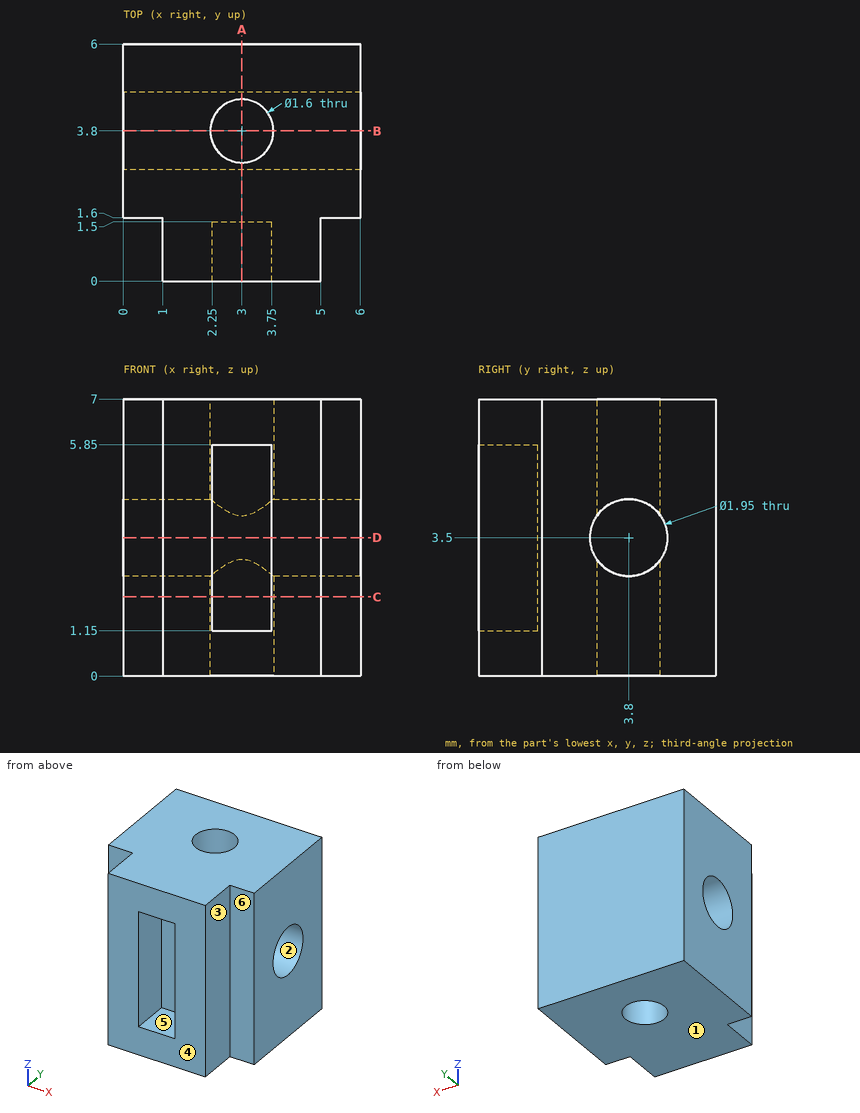
Design review of the part shown in the three views and the two pictorial views. Dimensions are in mm from the part's minimum x, y and z. A direction names the side the tool comes from. Round coordinates to 2 decimals unless told otherwise and drop trailing zeros. Order: outer loops, then holes, each group sorted by start corner. A loop starts at its lowest first (then second) coordinate and runs counter-clockwise, first axis right, second up.
Q1. Machinability: for the marked faces 4, 5 and 6, which of the approach directions +Z, -Z, +X, -X, +Y, -Y give a long, thin tool a straight path to every point of the face, cutting with its end or side? Answer none if there is none.
Findings below:
face 4: +Z, -Z, +X, -X, -Y
face 5: -Y
face 6: +Z, -Z, +X, -Y
Q2. We need section D-D, the plane z = 3.5. Give the boundary of the cut face in (x, y) (3 decimals).
Findings below:
outline: (0, 1.6) - (1, 1.6) - (1, 0) - (2.25, 0) - (2.25, 1.5) - (3.75, 1.5) - (3.75, 0) - (5, 0) - (5, 1.6) - (6, 1.6) - (6, 2.825) - (0, 2.825) - close; (0, 4.775) - (6, 4.775) - (6, 6) - (0, 6) - close
Q3. We need section C-C, the plane z = 2. Give the boundary of the cut face in (x, y), plus the area to 3 significant figures.
Findings below:
outline: (0, 1.6) - (1, 1.6) - (1, 0) - (2.25, 0) - (2.25, 1.5) - (3.75, 1.5) - (3.75, 0) - (5, 0) - (5, 1.6) - (6, 1.6) - (6, 6) - (0, 6) - close; hole circle Ø1.6 at (3, 3.8)
area: 28.5 mm2
Q4. Wall thickness on line 1 (Y direction, x = 3, z = 2.15); line 2 (Y direction, x = 4, z = 3.5) (3 decimals); line 3 (X direction, y = 1.45, z = 4.25): over which ranges is each line inside the solid? List them lowest first.
Findings below:
line 1: y = 1.5 to 3, 4.6 to 6
line 2: y = 0 to 2.825, 4.775 to 6
line 3: x = 1 to 2.25, 3.75 to 5
Q5. Insertion check: P1, Ø0.5, axis at y = 0.5, z = 4.5, coming from the +X side; P2, Ø0.5, axis at y = 0.5, z = 3.5, coming from the -X side; P3, Ø3, axis at x = 2, z = 5, coming from the -Y side; P4, Ø1.8, axis at y = 3.8, z = 3.5, coming from the +X side. Each pin has a flat end and moves straight along its axis. Give the tip position at first contact, or say it passes through.
Findings below:
P1: stops at x = 5
P2: stops at x = 1
P3: stops at y = 0
P4: passes through
Q6. Mouldability with a two-part tool opening along Z and no side actions: class the marked faces 1, 2 and 3 as pulls with the +Z half, pulls with the -Z half, needs draft (parallel to the pull), parting line crosses it, or undercut.
Findings below:
face 1: pulls with the -Z half
face 2: undercut
face 3: needs draft
Q7. We need section A-A, the plane x = 3. Give the boundary of the cut face in (y, z) (3 decimals).
Findings below:
outline: (0, 0) - (3, 0) - (3, 2.943) arc R0.975 cw to (3, 4.057) - (3, 7) - (0, 7) - (0, 5.85) - (1.5, 5.85) - (1.5, 1.15) - (0, 1.15) - close; (4.6, 0) - (6, 0) - (6, 7) - (4.6, 7) - (4.6, 4.057) arc R0.975 cw to (4.6, 2.943) - close
Q8. We need section B-B, the plane y = 3.8. Give the boundary of the cut face in (x, z) (3 decimals), plus the area to 3 significant figures.
Findings below:
outline: (0, 0) - (2.2, 0) - (2.2, 2.525) - (0, 2.525) - close; (0, 4.475) - (2.2, 4.475) - (2.2, 7) - (0, 7) - close; (3.8, 0) - (6, 0) - (6, 2.525) - (3.8, 2.525) - close; (3.8, 4.475) - (6, 4.475) - (6, 7) - (3.8, 7) - close
area: 22.2 mm2
